from build123d import *

# Parameters (mm, degrees)
SKETCH2_R = 0.381


with BuildPart() as part:
    # Sweep1: sweep along a path in Sketch3
    with BuildLine(Plane(origin=(0, 0, 0), x_dir=(0, 0, -1), z_dir=(1, 0, 0))) as sweep1_path:
        Line((0, 0), (0, 4))
        ThreePointArc((0, 4), (0.292893219, 4.707106781), (1, 5))
        Line((1, 5), (17, 5))
        ThreePointArc((17, 5), (17.707106781, 4.707106781), (18, 4))
        Line((18, 4), (18, 0))
    # Sketch2 → Sweep1 (sweep)
    with BuildSketch(Plane(origin=(0, 0, 0), x_dir=(1, 0, 0), z_dir=(0, 1, 0))):
        Circle(SKETCH2_R)
    sweep(path=sweep1_path.line)


solid = part.part
Work out the finished part from the listing and answer in its coordinate system (mm). Give positions to 0.01 mm unless a question says otherwise; leave off trailing zeros. Write each loop counter-clockwise with the first axis right and the second up, starting at its lowest first coordinate (ties: lowest second). Pieces come first, ordered by that corner, then holes.
Q1. Straight lines are drawn through the part: L1, parallel to Z at x = 0, y = 0.3; L2, parallel to Z at x = 0.2, y = 2.45; L3, parallel to Y at x = -0.2, z = -17.5. For each, find the intervals that lie inside material, in ascending order.
Answer:
L1: z = -18.38 to -17.62, -0.38 to 0.38
L2: z = -18.32 to -17.68, -0.32 to 0.32
L3: y = 4.45 to 5.23
Q2. The part is cut by section A-A on y = 2.7. Give the vertices of the cut face in (x, z), and give its area (3 significant figures).
Answer:
outline: circle Ø0.76 at (0, -18); circle Ø0.76 at (0, 0)
area: 0.912 mm2
Q3. The part is cut by section C-C on z = -10.25. Give the vertices of the cut face in (x, y).
Answer:
outline: circle Ø0.76 at (0, 5)
Q4. The part is cut by section B-B on x = 0. Give the vertices of the cut face in (y, z).
Answer:
outline: (0, -18.38) - (4, -18.38) arc R1.38 ccw to (5.38, -17) - (5.38, -1) arc R1.38 ccw to (4, 0.38) - (0, 0.38) - (0, -0.38) - (4, -0.38) arc R0.62 cw to (4.62, -1) - (4.62, -17) arc R0.62 cw to (4, -17.62) - (0, -17.62) - close
